Design review of the part built by this model. Coordinates are the model's own, in mm. A direction names the side the tool comes from. Give positions to 0.01 mm unless a question says otherwise; leave off trailing zeros. Write each loop counter-clockwise with the first axis right and the second up, starting at its lowest first coordinate (ties: lowest second). Pieces come first, ordered by that corner, then holes. Notation, with made-up numbers: (-37.5, 75.5) - (-21.5, 75.5) arc R30 cw to (-21.5, 100.5) - close; hole circle Ø8 at (40, 33). An arc over 180 degrees is marked (long way). Write each question's results on one line, items separated by ' | '. Start each with the question number.
Autodesk Inventor part; units mm, degrees
ref_plane "YZ Plane" through (0, 0, 0) normal (1, 0, 0) x (0, 1, 0)
ref_plane "XZ Plane" through (0, 0, 0) normal (0, 1, 0) x (-1, 0, 0)
ref_plane "XY Plane" through (0, 0, 0) normal (0, 0, 1) x (1, 0, 0)
sketch "Sketch1" plane through (0, 0, 0) normal (1, 0, 0) x (0, 0, -1)
  line L0 (76.417, -156.0446) -> (38.7716, -168.593)
  line L1 (38.7716, -168.593) -> (-87.6783, -168.593)
  line L2 (-87.6783, -168.593) -> (-87.6783, -123.2255)
  line L3 (-87.6783, -123.2255) -> (-32.6581, -109.7118)
  line L4 (-32.6581, -109.7118) -> (-32.6581, -129.9824)
  line L5 (-32.6581, -129.9824) -> (76.417, -129.9824)
  line L6 (76.417, -129.9824) -> (76.417, -156.0446)
  line L7 (-16.2486, -129.9824) -> (-16.2486, -7.8675)
  line L8 (-16.2486, -7.8675) -> (-37.4845, -7.8675)
  line L9 (-37.4845, -7.8675) -> (-37.4845, -28.1467)
  line L10 (-37.4845, -28.1467) -> (-91.5394, -22.8377)
  line L11 (-91.5394, -22.8377) -> (-91.5394, 23.4951)
  line L12 (-91.5394, 23.4951) -> (0, 23.4951)
  line L13 (0, 23.4951) -> (21.8795, 37.0088)
  arc A0 (38.3256, 14.8774) -> (21.8795, 37.0088) centre (29.1509, 25.2359) ccw
  line L14 (38.3256, 14.8774) -> (21.8883, 0.3187)
  line L15 (21.8883, 0.3187) -> (21.8795, -129.9824)
  line L16 (76.417, -129.9824) -> (76.417, -100.2282)
  line L17 (76.417, -100.2282) -> (46.4938, -100.2282)
  line L18 (46.4938, -100.2282) -> (46.4938, -129.9824)
  line L19 (46.4938, -129.9824) -> (76.417, -129.9824)
  point P0 (0, 0)
extrude "Extrusion1" add sketch "Sketch1" along normal mid plane 12.7 contours L0 L1 L2 L3 L4 L5 L6 | L5 L7 L8 L9 L10 L11 L12 L13 A0 L14 L15
extrude "Extrusion2" add sketch "Sketch1" along normal mid plane 31.75 contours L5 L18 L17 L16
sketch "Sketch2" plane through (15.875, -100.2282, -76.417) normal (0, 1, 0) x (-1, 0, 0)
  circle A0 centre (15.875, 13.936) radius 9.5136
  point P0 (15.875, 76.417)
extrude "Extrusion3" add sketch "Sketch2" along normal blind 98.425
sketch "Sketch3" plane through (0, -1.8032, -62.481) normal (0, 1, 0) x (1, 0, 0)
  circle A0 centre (0, 0) radius 25.4
  point P0 (0, -62.481)
  dimension "d6" = 50.8
extrude "Extrusion4" add sketch "Sketch3" along normal blind 180.34
sketch "Sketch4" plane through (6.35, 0, 0) normal (1, 0, 0) x (0, 0, -1)
  arc A0 (37.8876, 35.9665) -> (21.8795, 37.0088) centre (29.1509, 25.2359) ccw
  point P0 (0, 0)
  point P1 (22.8739, -26.7555)
hole "Hole1" at (6.35, 25.2359, -29.1509) direction (-1, 0, 0) diameter 12.7 end through all
properties part number "Sustitue Clamp"
Q1. Add section C-C on y = 10. State the section outline as (x, z) points, plus the area to 3 significant figures.
Q2. Add section D-D on z = 72. State the section outline as (x, y) points.
Q3. Add section A-A on z = 20.5. State the section outline as (x, y) points.
Q4. Insertion check: P1, Ø3, axis at x = 10.5, z = -62.5, coming from the -Y side; P2, Ø10, axis at x = 3.5, y = -58.5, coming from the -Z side; P3, Ø4, axis at x = 6.5, z = -55, coming from the -Y side. Each pin has a flat end and moves straight along its axis. Give the tip position at first contact, or say it passes through.
Q5. Machinability: for faces 1 (the face through (0, -129.982, 25)), 2 (the face through (0, 23.495, 46)), 3 (the face through (-15.875, -115, -61)), 4 (the face through (-7, -100.228, -55)), 5 (the face through (15.875, -115, -61)), which of the approach directions +Z, -Z, +X, -X, +Y, -Y give a long, thin tool a straight path to every point of the face, cutting with its end or side? Answer none if there is none.
Q6. For line 1 along Y through (x, z) = (-2, 19); line 2 along Y through (x, z) = (-18.5, -68); line 3 along X through (y, z) = (-52.5, 2), list the stretches that pass through material, from the lowest coordinate up. Write a range as [from, to].
Q7. The part is to be moulded in two halves that separate along Y. For faces 6 (the face through (0, -146, 87.678)), 7 (the face through (-11, -129.982, -61)), 8 (the face through (0, -18, 37.484)), say which applies: +Y half, -Y half, draft (parallel to the pull), parting line (faces both ways), or undercut.
Q8. Add section B-B on x = -3. Count the separate pieces of the cut face and the enclosed holes in it, plus the area to 3 significant figures.
Result:
1) outline: circle Ø50.8 at (0, -62.48); (-6.35, -32.82) - (6.35, -32.82) - (6.35, 91.54) - (-6.35, 91.54) - close | area: 3,610 mm²
2) outline: (-6.35, -168.59) - (6.35, -168.59) - (6.35, -119.37) - (-6.35, -119.37) - close; (-6.35, -24.76) - (6.35, -24.76) - (6.35, 23.5) - (-6.35, 23.5) - close
3) outline: (-6.35, -168.59) - (6.35, -168.59) - (6.35, -129.98) - (-6.35, -129.98) - close; (-6.35, -7.87) - (6.35, -7.87) - (6.35, 23.5) - (-6.35, 23.5) - close
4) P1: stops at y = -129.98 | P2: stops at z = -71.99 | P3: stops at y = -163.85
5) face 1: +X, -X | face 2: +Z, +X, -X, +Y | face 3: +Z, -Z, -X, -Y | face 4: none | face 5: +Z, -Z, +X, -Y
6) line 1: y = [-168.59, -129.98], [-7.87, 23.5] | line 2: y = [-1.8, 178.54] | line 3: x = [-6.35, 6.35]
7) face 6: draft | face 7: -Y half | face 8: undercut
8) separate pieces: 1 | enclosed holes: 2 | area: 28,300 mm²
